The model under review builds one solid part; all positions refer to its coordinate system, in mm. Face numbers are marked on the shaded views. A direction names the side the tool comes from. Coordinates: 2 decimals unless noted, no trailing zeros. Loops run counter-clockwise (first coordinate to the right, second up) from the corner with the lowest first, then second, coordinate; pieces in that order, holes last. Notation, with made-up numbers: (11.25, 19) - (27.25, 19) arc R15 cw to (27.25, 24) - close; hole circle Ø1 at (59, 34.25). An arc over 180 degrees is marked (long way). Answer in a Markdown table with one row per item. Add a question column.
(1) We need section A-A on x = 21. Write out the cut boundary in (y, z), plus the area to 3 significant figures.
(2) For line 1 along Z through (x, y) = (7, 0.25); line 2 along Z through (x, y) = (13.5, -4.25); line 3 along X through (y, z) = (3.5, -3), list the stretches that pass through material, from the lowest coordinate up.
(3) Machinability: for the marked faces 1 and 2, which of the approach directions +Z, -Z, +X, -X, +Y, -Y give a long, thin tool a straight path to every point of the face, cutting with its end or side? Answer none if there is none.
(4) For P1, Ø4, axis at x = 6.5, y = -3.5, coming from the +Z side; P2, Ø8, axis at x = 30.5, z = 0.5, coming from the -Y side; P3, Ø8, axis at x = 31, y = 2, coming from the -Z side, all flat-tipped, find the tip position at first contact; note any pin that passes through.
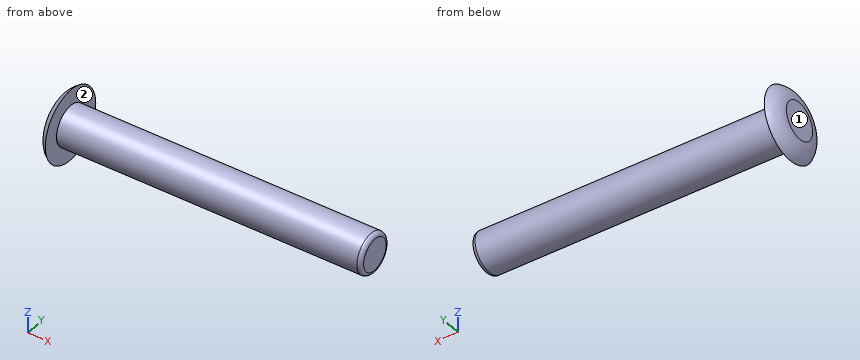
from build123d import *

# Parameters (mm, degrees)
F0_R     = 5
F2_DEPTH = 76.2
F1_R     = 9
F3_DEPTH = 2.5
F5_R     = 1


# Not quite as in the source:
# - a fillet or chamfer that OpenCascade refuses, or shapes differently, is made with other operations: its cross-section is extruded or revolved along the edge and cut away or added


with BuildPart() as f2:
    # F0 (on Right) → F2 (new body)
    with BuildSketch(Plane.YZ):
        Circle(F0_R)
    extrude(amount=F2_DEPTH)

    # F1 (on Right) → F3 (join)
    with BuildSketch(Plane.YZ):
        Circle(F1_R)
    extrude(amount=-F3_DEPTH)

    # F4: fillet of radius 5 on 1 edges, made by hand

    # F4_s1 → F4_t2 (revolve, cut)
    with BuildSketch(Plane.XY):
        with BuildLine():
            ThreePointArc((0, 9), (-1.8301270189, 7.1698729811), (-2.5, 4.6698729811))
            Line((-2.5, 4.6698729811), (-2.5, 9))
            Line((-2.5, 9), (0, 9))
        make_face()
    revolve(axis=Axis((-2.5, 0, 0), (1, 0, 0)), mode=Mode.SUBTRACT)

    # F5
    f5_edges = [f2.edges().sort_by_distance(p)[0] for p in [
        (76.2, -5, 0),
    ]]
    fillet(f5_edges, radius=F5_R)


solid = f2.part
Outcome:
| question | item | result |
|---|---|---|
| 1 | outline | circle Ø10 at (0, 0) |
| 1 | area | 78.5 mm² |
| 2 | line 1 | -4.99 to 4.99 |
| 2 | line 2 | -2.63 to 2.63 |
| 2 | line 3 | -2.5 to 75.99 |
| 3 | face 1 | +Z, -Z, -X, +Y, -Y |
| 3 | face 2 | +X |
| 4 | P1 | z = 4.77 |
| 4 | P2 | y = -5 |
| 4 | P3 | z = -5 |
